Geometry: final body of the model. Coordinates: model frame, mm. Face numbers are marked on the shaded views. A direction names the side the tool comes from. Give positions to 0.01 mm unless a question says otherwise; leave off trailing zeros. Write each loop counter-clockwise with the first axis right and the second up, starting at its lowest first coordinate (ties: lowest second). Pieces come first, ordered by that corner, then holes. Notation, with made-up numbers: (65.5, 60) -> (123.5, 60) arc R27 ccw to (123.5, 91) -> close; hole circle Ø11 at (29, 36). An arc over 180 degrees is marked (long way). Answer in a Markdown table with one row per item. Add a question column.
Item 1: Section query B-B on y = 7. Output: boundary loops of the cut face in (x, z), plus the area to 3 significant figures.
Item 2: Section query C-C on z = 8.5. Output: boundary loops of the cut face in (x, y).
Item 3: First-contact query: P1, Ø10, axis at x = -0.5, y = -7.5, coming from the +Z side; P2, Ø12, axis at x = 3, y = 5, coming from the -Z side; P3, Ø4.5, axis at y = 5, z = 4.5, coming from the -X side; P4, Ø4, axis at x = -2.5, y = 7, coming from the +Z side. Flat tips, straight axial feed; report the tip coordinate or a pass-through.
Item 4: Section query D-D on y = 2.5. Output: boundary loops of the cut face in (x, z).
Item 5: Access query for the marked faces 1, 2 and 3. Directions: +Z, -Z, +X, -X, +Y, -Y. A direction counts if a zero-diameter tool reaches every point of the face in a straight line with its end or side. Return the directions, or none.
Item 6: Material intervals for probe 1 along Z at (x, y) = (-8.75, -6.25); probe 2 along X at (y, z) = (5.75, 5.75); probe 3 along Y at (x, z) = (2.5, 2.5), sorted ascending. Write a range as from..to.
Item 7: Section query A-A on x = 4.25. Output: boundary loops of the cut face in (y, z).
```python
from build123d import *

# Parameters (mm, degrees)
F0_W     = 20
F0_H     = 25
F1_DEPTH = 1
F3_DEPTH = 8


with BuildPart() as f1:
    # F0 (on Top) → F1 (new body)
    with BuildSketch(Plane.XY):
        Rectangle(F0_W, F0_H)
    extrude(amount=F1_DEPTH)

    # F2 (on Right) → F3 (join, symmetric)
    with BuildSketch(Plane.YZ):
        with BuildLine():
            Line((9.680679, 4.11431), (2.951698, 9.035775))
            ThreePointArc((2.951698, 9.035775), (0, 10), (-2.951698, 9.035775))
            Line((-2.951698, 9.035775), (-9.680679, 4.11431))
            ThreePointArc((-9.680679, 4.11431), (-10.283446, 3.405163), (-10.5, 2.5))
            Line((-10.5, 2.5), (-10.5, 1))
            Line((-10.5, 1), (10.5, 1))
            Line((10.5, 1), (10.5, 2.5))
            ThreePointArc((10.5, 2.5), (10.283446, 3.405163), (9.680679, 4.11431))
        make_face()
    extrude(amount=F3_DEPTH, both=True)


solid = f1.part
```
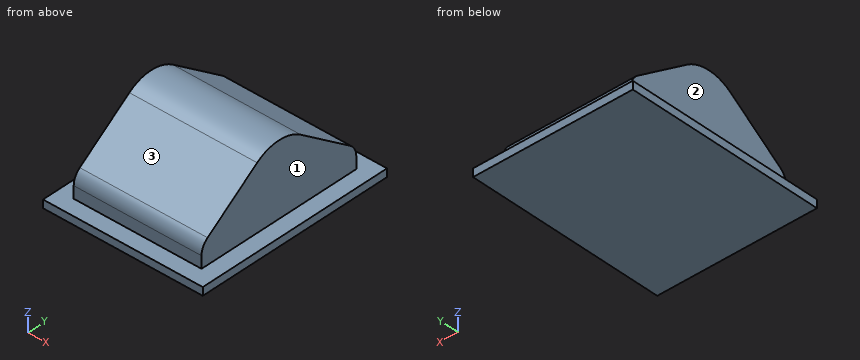
Findings below:
| question | item | result |
|---|---|---|
| 1 | outline | (-10, 0) -> (10, 0) -> (10, 1) -> (8, 1) -> (8, 6.07) -> (-8, 6.07) -> (-8, 1) -> (-10, 1) -> close |
| 1 | area | 101 mm^2 |
| 2 | outline | (-8, -3.68) -> (8, -3.68) -> (8, 3.68) -> (-8, 3.68) -> close |
| 3 | P1 | stops at z = 9.33 |
| 3 | P2 | stops at z = 0 |
| 3 | P3 | stops at x = -8 |
| 3 | P4 | stops at z = 7.54 |
| 4 | outline | (-10, 0) -> (10, 0) -> (10, 1) -> (8, 1) -> (8, 9.33) -> (-8, 9.33) -> (-8, 1) -> (-10, 1) -> close |
| 5 | face 1 | +Z, +X, +Y, -Y |
| 5 | face 2 | +Z, -X, +Y, -Y |
| 5 | face 3 | +Z, +X, -X, -Y |
| 6 | probe 1 | z = 0..1 |
| 6 | probe 2 | x = -8..8 |
| 6 | probe 3 | y = -10.5..10.5 |
| 7 | outline | (-12.5, 0) -> (12.5, 0) -> (12.5, 1) -> (10.5, 1) -> (10.5, 2.5) arc R2 ccw to (9.68, 4.11) -> (2.95, 9.04) arc R5 ccw to (-2.95, 9.04) -> (-9.68, 4.11) arc R2 ccw to (-10.5, 2.5) -> (-10.5, 1) -> (-12.5, 1) -> close |
